```python
from build123d import *

# Parameters (mm, degrees)
SKETCH1_R           = 40
BOSS_EXTRUDE1_DEPTH = 2
SKETCH2_W           = 4.6
SKETCH2_H           = 2.6
BOSS_EXTRUDE2_DEPTH = 4
SKETCH3_R           = 36
SKETCH3_R_2         = 34
BOSS_EXTRUDE3_DEPTH = 2
FILLET2_R           = 1
CUT_EXTRUDE1_DEPTH  = 2
SKETCH5_W           = 4.6
SKETCH5_H           = 2.6
SKETCH5_W_2         = 4.3
SKETCH5_H_2         = 2.3
CUT_EXTRUDE2_DEPTH  = 4
FILLET3_R           = 1.5


with BuildPart() as part:
    # Sketch1 → Boss-Extrude1 (new body)
    with BuildSketch(Plane(origin=(0, 0, 0), x_dir=(1, 0, 0), z_dir=(0, 1, 0))):
        with Locations(Location((0, 0, 0), (0, 0, 270))):
            Circle(SKETCH1_R)
    extrude(amount=BOSS_EXTRUDE1_DEPTH)

    # Sketch2 → Boss-Extrude2 (add)
    with BuildSketch(Plane(origin=(0, 2, 0), x_dir=(1, 0, 0), z_dir=(0, 1, 0))):
        with Locations((0, 35.9)):
            Rectangle(SKETCH2_W, SKETCH2_H)
        Polygon((34.668563319, 13.682862178), (36.090041493, 9.308002203), (33.617294551, 8.504558018), (32.195816377, 12.879417993), align=None)
        Polygon((23.726350472, -28.74352611), (20.004872298, -31.447338271), (18.476630642, -29.343894086), (22.198108816, -26.640081925), align=None)
        Polygon((-20.004872298, -31.447338271), (-23.726350472, -28.74352611), (-22.198108816, -26.640081925), (-18.476630642, -29.343894086), align=None)
        Polygon((-36.090041493, 9.308002203), (-34.668563319, 13.682862178), (-32.195816377, 12.879417993), (-33.617294551, 8.504558018), align=None)
    extrude(amount=BOSS_EXTRUDE2_DEPTH)

    # Sketch3 → Boss-Extrude3 (add)
    with BuildSketch(Plane.XZ):
        with Locations(Location((0, 0, 0), (0, 0, 90))):
            Circle(SKETCH3_R)
        with Locations(Location((0, 0, 0), (0, 0, 270))):
            Circle(SKETCH3_R_2, mode=Mode.SUBTRACT)
    extrude(amount=BOSS_EXTRUDE3_DEPTH)

    # Fillet2
    fillet2_edges = [part.edges().sort_by_distance(p)[0] for p in [
        (0, -2, -36),
        (0, -2, 34),
    ]]
    fillet(fillet2_edges, radius=FILLET2_R - 0.0001)  # a hair under: the kernel refuses the full size

    # Sketch4 → Cut-Extrude1 (cut)
    with BuildSketch(Plane.XZ):
        Polygon((-1.5, -40), (-1.5, -1.5), (-40, -1.5), (-40, 1.5), (-1.5, 1.5), (-1.5, 40), (1.5, 40), (1.5, 1.5), (40, 1.5), (40, -1.5), (1.5, -1.5), (1.5, -40), align=None)
    extrude(amount=CUT_EXTRUDE1_DEPTH, mode=Mode.SUBTRACT)

    # Sketch5 → Cut-Extrude2 (cut)
    # profile 1 of 5: a face of its own
    with BuildSketch(Plane(origin=(0, 6, 0), x_dir=(1, 0, 0), z_dir=(0, 1, 0))):
        Polygon((34.668563319, 13.682862178), (32.195816377, 12.879417993), (33.617294551, 8.504558018), (36.090041493, 9.308002203), align=None)
        Polygon((34.572257391, 13.493851152), (32.384827403, 12.783112065), (33.713600479, 8.693569044), (35.901030467, 9.404308132), align=None, mode=Mode.SUBTRACT)
    # profile 2 of 5: a face of its own
    with BuildSketch(Plane(origin=(0, 6, 0), x_dir=(1, 0, 0), z_dir=(0, 1, 0))):
        with Locations((0, 35.9)):
            Rectangle(SKETCH5_W, SKETCH5_H)
        with Locations((0, 35.9)):
            Rectangle(SKETCH5_W_2, SKETCH5_H_2, mode=Mode.SUBTRACT)
    # profile 3 of 5: a face of its own
    with BuildSketch(Plane(origin=(0, 6, 0), x_dir=(1, 0, 0), z_dir=(0, 1, 0))):
        Polygon((23.726350472, -28.74352611), (22.198108816, -26.640081925), (18.476630642, -29.343894086), (20.004872298, -31.447338271), align=None)
        Polygon((23.516830135, -28.710341349), (22.164924055, -26.849602262), (18.686150979, -29.377078847), (20.03805706, -31.237817934), align=None, mode=Mode.SUBTRACT)
    # profile 4 of 5: a face of its own
    with BuildSketch(Plane(origin=(0, 6, 0), x_dir=(1, 0, 0), z_dir=(0, 1, 0))):
        Polygon((-20.004872298, -31.447338271), (-18.476630642, -29.343894086), (-22.198108816, -26.640081925), (-23.726350472, -28.74352611), align=None)
        Polygon((-20.03805706, -31.237817934), (-18.686150979, -29.377078847), (-22.164924055, -26.849602262), (-23.516830135, -28.710341349), align=None, mode=Mode.SUBTRACT)
    # profile 5 of 5: a face of its own
    with BuildSketch(Plane(origin=(0, 6, 0), x_dir=(1, 0, 0), z_dir=(0, 1, 0))):
        Polygon((-36.090041493, 9.308002203), (-33.617294551, 8.504558018), (-32.195816377, 12.879417993), (-34.668563319, 13.682862178), align=None)
        Polygon((-35.901030467, 9.404308132), (-33.713600479, 8.693569044), (-32.384827403, 12.783112065), (-34.572257391, 13.493851152), align=None, mode=Mode.SUBTRACT)
    extrude(amount=-CUT_EXTRUDE2_DEPTH, mode=Mode.SUBTRACT)

    # Fillet3
    fillet3_edges = [part.edges().sort_by_distance(p)[0] for p in [
        (-2.15, 6, -35.9),
        (2.15, 6, -35.9),
        (33.478542397, 6, -13.138481608),
        (34.807315473, 6, -9.048938588),
        (22.840877095, 6, 27.779971806),
        (19.362104019, 6, 30.30744839),
        (-19.362104019, 6, 30.30744839),
        (-22.840877095, 6, 27.779971806),
        (-34.807315473, 6, -9.048938588),
        (-33.478542397, 6, -13.138481608),
    ]]
    fillet(fillet3_edges, radius=FILLET3_R)


solid = part.part
```
Here's how the part is built. I have some questions about the finished solid (model axes, mm). A direction names the side the tool comes from. Give positions to 0.01 mm unless a question says otherwise; leave off trailing zeros. Order: outer loops, then holes, each group sorted by start corner. A loop starts at its lowest first (then second) coordinate and runs counter-clockwise, first axis right, second up. Notation, with made-up numbers: M 84.5,62 L 109.5,62 A11 ccw 109.5,71 Z; hole C -9.75,77 d5. An arc over 180 degrees is marked long. Use a Markdown table: item, result. Add a question column.
1. Suppose I cut it at A-A (z = 0). List the corners of the cut face in (x, y) for me.
2. On a 3-axis mill with a long thin cutter (end or side, diameter ignored), from which of +Z, -Z, +X, -X, +Y, -Y can I reach the whole of each face in a straight line? I mean faces 1 (the flat face through (0, 4, -37.05)), 2 (the flat face through (0, 4, -34.75)), 3 (the flat face through (35, -1, 1.5)), 4 (the cylindrical face through (23.79, -0.49, -24.29)). Say none if no direction works.
3. I need wall thicknesses on probe 1 along Y at (x, z) = (7.5, -21); probe 2 along X at (y, z) = (2.75, -10.5); probe 3 along X at (y, z) = (5.5, -10). Which ranges of each line are inside material? Lowest first, please. Write a range as from..to.
4. For pin 1 Ø24 at (x, z) = (8, 0) entering from -Y; pin 2 Ø2 at (x, z) = (12.5, 7) entering from +Y; pin 3 Ø3 at (y, z) = (1.5, 7) entering from +X, each with a flat end and sliding along its axis, tell me the tip position at first contact or that it passes through.
Results list:
| question | item | result |
|---|---|---|
| 1 | outline | M -40,0 L 40,0 L 40,2 L -40,2 Z |
| 2 | face 1 | -Z, +X, -X, +Y |
| 2 | face 2 | +Z, +X, -X, +Y |
| 2 | face 3 | +X, -X, -Y |
| 2 | face 4 | -Y |
| 3 | probe 1 | y = 0..2 |
| 3 | probe 2 | x = -35.55..-33.13, 33.13..35.55 |
| 3 | probe 3 | x = -35.71..-33.29, 33.29..35.71 |
| 4 | pin 1 | stops at y = 0 |
| 4 | pin 2 | stops at y = 2 |
| 4 | pin 3 | stops at x = 39.62 |
